from build123d import *

# Parameters (mm, degrees)
SKETCH_2_R          = 1.5
EXTRUDE_1_DEPTH     = 2
SKETCH_3_W          = 2
SKETCH_3_H          = 20
SKETCH_3_W_2        = 3.5
EXTRUDE_2_DEPTH     = 55
SKETCH_9_R          = 6
CUT_EXTRUDE_1_DEPTH = 87
SKETCH_7_R          = 6
SKETCH_7_R_2        = 3.3
EXTRUDE_3_DEPTH     = 2
SKETCH_10_R         = 3.3
EXTRUDE_4_DEPTH     = 1.5
SKETCH_11_W         = 68
SKETCH_11_H         = 20
SKETCH_11_R         = 1.5
SKETCH_11_R_2       = 1.498871695
EXTRUDE_5_DEPTH     = 1
FILLET_6_R          = 5
FILLET_7_R          = 5
FILLET_8_R          = 5


with BuildPart() as part:
    # 스케치2 → 보스-돌출1 (new body)
    with BuildSketch(Plane(origin=(0, 0, 0), x_dir=(1, 0, 0), z_dir=(0, 1, 0))):
        Polygon((35, -10), (-35, -10), (-35, 10), (35, 10), (38.5, 10), (38.5, -10), align=None)
        with Locations((-15, 5)):
            Circle(SKETCH_2_R, mode=Mode.SUBTRACT)
        with Locations((-5, 5)):
            Circle(SKETCH_2_R, mode=Mode.SUBTRACT)
        with Locations((-15, -5)):
            Circle(SKETCH_2_R, mode=Mode.SUBTRACT)
        with Locations((-5, -5)):
            Circle(SKETCH_2_R, mode=Mode.SUBTRACT)
        with Locations((15, -5)):
            Circle(SKETCH_2_R, mode=Mode.SUBTRACT)
        with Locations((5, -5)):
            Circle(SKETCH_2_R, mode=Mode.SUBTRACT)
        with Locations((5, 5)):
            Circle(SKETCH_2_R, mode=Mode.SUBTRACT)
        with Locations((15, 5)):
            Circle(SKETCH_2_R, mode=Mode.SUBTRACT)
    extrude(amount=EXTRUDE_1_DEPTH)

    # 스케치3 → 보스-돌출2 (add)
    with BuildSketch(Plane(origin=(0, 2, 0), x_dir=(1, 0, 0), z_dir=(0, 1, 0))):
        with Locations((-34, 0)):
            Rectangle(SKETCH_3_W, SKETCH_3_H)
        with Locations((36.75, 0)):
            Rectangle(SKETCH_3_W_2, SKETCH_3_H)
    extrude(amount=EXTRUDE_2_DEPTH)

    # 스케치9 → 컷-돌출1 (cut)
    with BuildSketch(Plane(origin=(38.5, 0, 0), x_dir=(0, 0, -1), z_dir=(1, 0, 0))):
        with BuildLine():
            Line((10, 57), (0, 57))
            ThreePointArc((0, 57), (7.071067812, 54.071067812), (10, 47))
            Line((10, 47), (10, 57))
        make_face()
        with BuildLine():
            Line((-10, 57), (-10, 47))
            ThreePointArc((-10, 47), (-7.071067812, 54.071067812), (0, 57))
            Line((0, 57), (-10, 57))
        make_face()
        with Locations((0, 47)):
            Circle(SKETCH_9_R)
    extrude(amount=-CUT_EXTRUDE_1_DEPTH, mode=Mode.SUBTRACT)

    # 스케치7 → 보스-돌출3 (add)
    with BuildSketch(Plane.ZY.offset(35)):
        with Locations((0, 47)):
            Circle(SKETCH_7_R)
        with Locations((0, 47)):
            Circle(SKETCH_7_R_2, mode=Mode.SUBTRACT)
    extrude(amount=-EXTRUDE_3_DEPTH)

    # 스케치10 → 보스-돌출4 (add)
    with BuildSketch(Plane.ZY.offset(35)):
        with BuildLine():
            ThreePointArc((-10, 47), (0, 57), (10, 47))
            Line((10, 47), (10, 0))
            Line((10, 0), (-10, 0))
            Line((-10, 0), (-10, 47))
        make_face()
        with Locations((0, 47)):
            Circle(SKETCH_10_R, mode=Mode.SUBTRACT)
    extrude(amount=EXTRUDE_4_DEPTH)

    # 스케치11 → 보스-돌출5 (add)
    with BuildSketch(Plane(origin=(0, 2, 0), x_dir=(1, 0, 0), z_dir=(0, 1, 0))):
        with Locations((1, 0)):
            Rectangle(SKETCH_11_W, SKETCH_11_H)
        with Locations((-15, 5)):
            Circle(SKETCH_11_R, mode=Mode.SUBTRACT)
        with Locations((-5, 5)):
            Circle(SKETCH_11_R, mode=Mode.SUBTRACT)
        with Locations((5, 5)):
            Circle(SKETCH_11_R, mode=Mode.SUBTRACT)
        with Locations((15, 5)):
            Circle(SKETCH_11_R, mode=Mode.SUBTRACT)
        with Locations((15, -5)):
            Circle(SKETCH_11_R, mode=Mode.SUBTRACT)
        with Locations((5, -5)):
            Circle(SKETCH_11_R, mode=Mode.SUBTRACT)
        with Locations((-5, -5)):
            Circle(SKETCH_11_R, mode=Mode.SUBTRACT)
        with Locations((-15, -5)):
            Circle(SKETCH_11_R_2, mode=Mode.SUBTRACT)
    extrude(amount=EXTRUDE_5_DEPTH)

    # 필렛6
    fillet_6_edges = [part.edges().sort_by_distance(p)[0] for p in [
        (-33, 3, 0),
    ]]
    fillet(fillet_6_edges, radius=FILLET_6_R)

    # 필렛7
    fillet_7_edges = [part.edges().sort_by_distance(p)[0] for p in [
        (35, 3, 0),
    ]]
    fillet(fillet_7_edges, radius=FILLET_7_R)

    # 필렛8
    fillet_8_edges = [part.edges().sort_by_distance(p)[0] for p in [
        (-36.5, 0, 0),
        (38.5, 0, 0),
    ]]
    fillet(fillet_8_edges, radius=FILLET_8_R)


solid = part.part
Here's how the part is built. I have some questions about the finished solid (model axes, mm). A direction names the side the tool comes from. Give positions to 0.01 mm unless a question says otherwise; leave off trailing zeros. Order: outer loops, then holes, each group sorted by start corner. A loop starts at its lowest first (then second) coordinate and runs counter-clockwise, first axis right, second up. Notation, with made-up numbers: (48, 79) -> (93, 79) arc R7 cw to (93, 83) -> close; hole circle Ø5 at (66.25, -10.5). An arc over 180 degrees is marked (long way). One line per item, written item: value. Start each with the question number.
1. Imagine slicing it at B-B, the plane y = 28. List the corners of the cut face in (x, z) for me, plus the area to 3 significant figures.
2. Imagine slicing it at D-D, the plane y = 49. List the corners of the cut face in (x, z) for me.
3. Imagine slicing it at C-C, the plane z = -5. Count the separate pieces of the cut face and the enclosed holes in it, plus the area to 3 significant figures.
4. We'd pull the mould along X, two halves only. Please class faces 3 (the face through (38.5, 31, 0)), 4 (the face through (36.774, 41.143, 1.301)), 5 (the face through (-35, 1.43, -0.14)), 6 (the face through (13.5, 1.48, 4.93)): released by +X, released by -X, zero draft, split by the parting line, or undercut.
5. Imagine slicing it at A-A, the plane x = 15. List the corners of the cut face in (y, z) for me.
6. Will this pin go through, and if not, where does the flat tip stop? pin 1 Ø10 at (x, z) = (0, -4.5) entering from +Y.
7. For faces 1 (the face through (1, 3, 0)), 2 (the face through (37.07, 1.5, 0.14)), which set-ups out of +Z, -Z, +X, -X, +Y, -Y let a thin tool reach every point of the face, with its end or its side?
8. I need wall thicknesses on probe 1 along Z at (x, y) = (15, 1.2); probe 2 along X at (y, z) = (52, -8.25); probe 3 along X at (y, z) = (2.2, -5). Which ranges of each line are inside material? Lowest first, please. Write a range as from..to.
Values follow:
1. outline: (-36.5, -10) -> (-33, -10) -> (-33, 10) -> (-36.5, 10) -> close; (35, -10) -> (38.5, -10) -> (38.5, 10) -> (35, 10) -> close
1. area: 140 mm2
2. outline: (-36.5, -9.8) -> (-33, -9.8) -> (-33, -2.62) -> (-36.5, -2.62) -> close; (-36.5, 2.62) -> (-33, 2.62) -> (-33, 9.8) -> (-36.5, 9.8) -> close; (35, -9.8) -> (38.5, -9.8) -> (38.5, -5.66) -> (35, -5.66) -> close; (35, 5.66) -> (38.5, 5.66) -> (38.5, 9.8) -> (35, 9.8) -> close
3. separate pieces: 6
3. enclosed holes: 0
3. area: 534 mm2
4. face 3: released by +X
4. face 4: zero draft
4. face 5: released by -X
4. face 6: undercut
5. outline: (0, -10) -> (3, -10) -> (3, -6.5) -> (0, -6.5) -> close; (0, -3.5) -> (3, -3.5) -> (3, 3.5) -> (0, 3.5) -> close; (0, 6.5) -> (3, 6.5) -> (3, 10) -> (0, 10) -> close
6. pin 1: stops at y = 3
7. face 1: +Z, -Z, +Y
7. face 2: +Z, -Z, +X, -Y
8. probe 1: z = -10..-6.5, -3.5..3.5, 6.5..10
8. probe 2: x = -36.5..-33, 35..38.5
8. probe 3: x = -35.64..-16.5, -13.5..-6.5, -3.5..3.5, 6.5..13.5, 16.5..37.64
